Source: CAD feature listing. Evaluate the final solid. Frame: model axes, mm. Face numbers are marked on the shaded views. A direction names the side the tool comes from. Give positions to 0.01 mm unless a question says otherwise; leave off trailing zeros. Loops run counter-clockwise (first coordinate to the right, second up) from the corner with the lowest first, then second, coordinate; pieces in that order, holes last. Notation, with made-up numbers: M -33.75,6.5 L -3.75,6.5 A23 cw -3.75,29.5 Z; hole C -38,7.25 d5. An arc over 180 degrees is marked long. Answer in a Markdown table with one row per item.
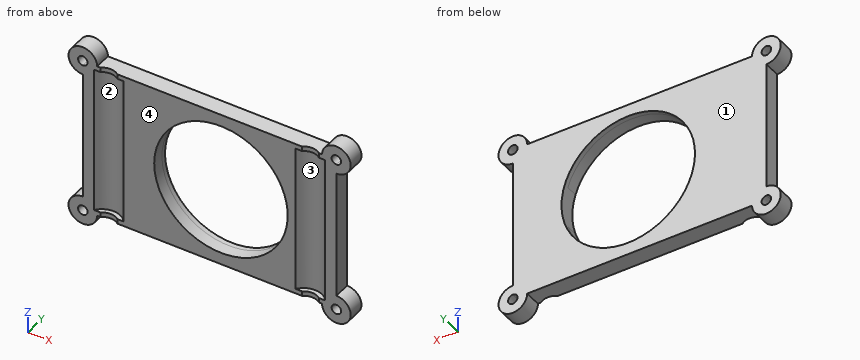
```python
from build123d import *
from build123d.topology import SkipClean

# Parameters (mm, degrees)
SKETCH1_W               = 21.76
SKETCH1_H               = 66
SKETCH1_W_2             = 62.8
BOSS_EXTRUDE1_DEPTH     = 10
SKETCH1_5_W             = 62.8
SKETCH1_5_H             = 66
CUT_EXTRUDE1_DEPTH      = 5
SKETCH3_R               = 7.65
SKETCH3_R_2             = 5.75
CUT_EXTRUDE2_DEPTH      = 62
CUT_EXTRUDE3_DEPTH      = 84.797288739
CUT_EXTRUDE3_DEPTH_BACK = 84.797288739
SKETCH3_3_R             = 5.75
BOSS_EXTRUDE2_DEPTH     = 10
CUT_EXTRUDE4_DEPTH      = 72.560503073
SKETCH5_R               = 28
CUT_EXTRUDE5_DEPTH      = 72.560503073
BOSS_EXTRUDE3_DEPTH     = 5
CUT_EXTRUDE6_START      = -3
CUT_EXTRUDE6_DEPTH      = 3


with BuildPart() as part:
    # Sketch1 → Boss-Extrude1 (new body)
    with BuildSketch(Plane(origin=(0, 0, 0), x_dir=(1, 0, 0), z_dir=(0, 1, 0))):
        with Locations((-42.28, 0)):
            Rectangle(SKETCH1_W, SKETCH1_H)
        Rectangle(SKETCH1_W_2, SKETCH1_H)
        with Locations((42.28, 0)):
            Rectangle(SKETCH1_W, SKETCH1_H)
    extrude(amount=BOSS_EXTRUDE1_DEPTH)

    # Sketch1<5> → Cut-Extrude1 (cut)
    with BuildSketch(Plane(origin=(0, 0, 0), x_dir=(1, 0, 0), z_dir=(0, 1, 0))):
        Rectangle(SKETCH1_5_W, SKETCH1_5_H)
    extrude(amount=CUT_EXTRUDE1_DEPTH, mode=Mode.SUBTRACT)

    # Sketch3 → Cut-Extrude2 (cut)
    # profile 1 of 4: a face of its own
    with BuildSketch(Plane.XY.offset(31)):
        with Locations((-42.25, -4.5)):
            Circle(SKETCH3_R)
        with Locations((-42.25, -4.5)):
            Circle(SKETCH3_R_2, mode=Mode.SUBTRACT)
    # profile 2 of 4: a face of its own
    with BuildSketch(Plane.XY.offset(31)):
        with Locations((-42.25, -4.5)):
            Circle(SKETCH3_R_2)
    # profile 3 of 4: a face of its own
    with BuildSketch(Plane.XY.offset(31)):
        with Locations((42.31, -4.5)):
            Circle(SKETCH3_R)
        with Locations((42.31, -4.5)):
            Circle(SKETCH3_R_2, mode=Mode.SUBTRACT)
    # profile 4 of 4: a face of its own
    with BuildSketch(Plane.XY.offset(31)):
        with Locations((42.31, -4.5)):
            Circle(SKETCH3_R_2)
    extrude(amount=-CUT_EXTRUDE2_DEPTH, mode=Mode.SUBTRACT)

    # Sketch3<3> → Cut-Extrude3 (cut, two sides: drawn at the far end of the back side and taken through both)
    with BuildSketch(Plane.XY.offset(31).offset(-CUT_EXTRUDE3_DEPTH_BACK)):
        with Locations((42.31, -4.5)):
            Circle(SKETCH3_3_R)
        with Locations((-42.25, -4.5)):
            Circle(SKETCH3_3_R)
    extrude(amount=CUT_EXTRUDE3_DEPTH + CUT_EXTRUDE3_DEPTH_BACK, mode=Mode.SUBTRACT)

    # Sketch4 → Boss-Extrude2 (add)
    with BuildSketch(Plane.XZ):
        with BuildLine():
            Line((-51.16, 33), (-47.16, 33))
            ThreePointArc((-47.16, 33), (-57.402640687, 37.242640687), (-53.16, 27))
            Line((-53.16, 27), (-53.16, 31))
            ThreePointArc((-53.16, 31), (-54.574213562, 34.414213562), (-51.16, 33))
        make_face()
        with BuildLine():
            ThreePointArc((-53.16, -27), (-57.402640687, -37.242640687), (-47.16, -33))
            Line((-47.16, -33), (-51.16, -33))
            ThreePointArc((-51.16, -33), (-54.574213562, -34.414213562), (-53.16, -31))
            Line((-53.16, -31), (-53.16, -27))
        make_face()
        with BuildLine():
            ThreePointArc((47.16, -33), (57.402640687, -37.242640687), (53.16, -27))
            Line((53.16, -27), (53.16, -31))
            ThreePointArc((53.16, -31), (54.574213562, -34.414213562), (51.16, -33))
            Line((51.16, -33), (47.16, -33))
        make_face()
        with BuildLine():
            ThreePointArc((53.16, 27), (57.402640687, 37.242640687), (47.16, 33))
            Line((47.16, 33), (51.16, 33))
            ThreePointArc((51.16, 33), (54.574213562, 34.414213562), (53.16, 31))
            Line((53.16, 31), (53.16, 27))
        make_face()
    extrude(amount=-BOSS_EXTRUDE2_DEPTH)

    # Sketch4<3> → Cut-Extrude4 (cut, through all)
    with SkipClean():  # the faces are left unmerged after this step: merging them gives an invalid solid
        with BuildSketch(Plane.XZ):
            with BuildLine():
                ThreePointArc((51.16, 33), (51.745786438, 31.585786438), (53.16, 31))
                Line((53.16, 31), (53.16, 33))
                Line((53.16, 33), (51.16, 33))
            make_face()
            with BuildLine():
                Line((53.16, 33), (53.16, 31))
                ThreePointArc((53.16, 31), (54.574213562, 31.585786438), (55.16, 33))
                ThreePointArc((55.16, 33), (53.16, 35), (51.16, 33))
                Line((51.16, 33), (53.16, 33))
            make_face()
            with BuildLine():
                ThreePointArc((55.16, -33), (54.574213562, -31.585786438), (53.16, -31))
                Line((53.16, -31), (53.16, -33))
                Line((53.16, -33), (51.16, -33))
                ThreePointArc((51.16, -33), (53.16, -35), (55.16, -33))
            make_face()
            with BuildLine():
                Line((53.16, -33), (53.16, -31))
                ThreePointArc((53.16, -31), (51.745786438, -31.585786438), (51.16, -33))
                Line((51.16, -33), (53.16, -33))
            make_face()
            with BuildLine():
                ThreePointArc((-53.16, -31), (-54.574213562, -34.414213562), (-51.16, -33))
                Line((-51.16, -33), (-53.16, -33))
                Line((-53.16, -33), (-53.16, -31))
            make_face()
            with BuildLine():
                Line((-53.16, -33), (-51.16, -33))
                ThreePointArc((-51.16, -33), (-51.745786438, -31.585786438), (-53.16, -31))
                Line((-53.16, -31), (-53.16, -33))
            make_face()
            with BuildLine():
                ThreePointArc((-53.16, 31), (-51.745786438, 31.585786438), (-51.16, 33))
                Line((-51.16, 33), (-53.16, 33))
                Line((-53.16, 33), (-53.16, 31))
            make_face()
            with BuildLine():
                Line((-53.16, 33), (-51.16, 33))
                ThreePointArc((-51.16, 33), (-54.574213562, 34.414213562), (-53.16, 31))
                Line((-53.16, 31), (-53.16, 33))
            make_face()
        extrude(amount=-CUT_EXTRUDE4_DEPTH, mode=Mode.SUBTRACT)

    # Sketch5 → Cut-Extrude5 (cut, through all)
    with SkipClean():  # the faces are left unmerged after this step: merging them gives an invalid solid
        with BuildSketch(Plane(origin=(0, 10, 0), x_dir=(1, 0, 0), z_dir=(0, 1, 0))):
            with Locations(Location((4.77, 0, 0), (0, 0, 270))):
                Circle(SKETCH5_R)
        extrude(amount=-CUT_EXTRUDE5_DEPTH, mode=Mode.SUBTRACT)

    # Sketch6 → Boss-Extrude3 (add)
    with SkipClean():  # the faces are left unmerged after this step: merging them gives an invalid solid
        with BuildSketch(Plane.XZ.offset(-5)):
            with BuildLine():
                Line((31.4, -33), (31.4, -8.651190669))
                ThreePointArc((31.4, -8.651190669), (-23.23, 0), (31.4, 8.651190669))
                Line((31.4, 8.651190669), (31.4, 33))
                Line((31.4, 33), (-31.4, 33))
                Line((-31.4, 33), (-31.4, -33))
                Line((-31.4, -33), (31.4, -33))
            make_face()
        extrude(amount=BOSS_EXTRUDE3_DEPTH)

    # Sketch8 → Cut-Extrude6 (cut)
    with SkipClean():  # the faces are left unmerged after this step: merging them gives an invalid solid
        with BuildSketch(Plane(origin=(0, 10, 0), x_dir=(1, 0, 0), z_dir=(0, 1, 0)).offset(CUT_EXTRUDE6_START)):
            with BuildLine():
                Line((-53.16, 27), (-53.16, -27))
                ThreePointArc((-53.16, -27), (-57.402640687, -37.242640687), (-47.16, -33))
                Line((-47.16, -33), (47.16, -33))
                ThreePointArc((47.16, -33), (57.402640687, -37.242640687), (53.16, -27))
                Line((53.16, -27), (53.16, 27))
                ThreePointArc((53.16, 27), (57.402640687, 37.242640687), (47.16, 33))
                Line((47.16, 33), (-47.16, 33))
                ThreePointArc((-47.16, 33), (-57.402640687, 37.242640687), (-53.16, 27))
            make_face()
        extrude(amount=CUT_EXTRUDE6_DEPTH, mode=Mode.SUBTRACT)


solid = part.part
```
Q1. Reachability of the marked faces 3 and 4 from +Z, -Z, +X, -X, +Y, -Y: full face, straight path, thin tool, end or side. Return the list, or none.
Values follow:
| item | result |
|---|---|
| face 3 | -Y |
| face 4 | +Z, -Z, +X, -X, -Y |
Q2. Section query B-B (x = 4.77). Output: boundary loops of the cut face in (y, z).
Values follow:
| item | result |
|---|---|
| outline | M 0,-33 L 7,-33 L 7,-28 L 0,-28 Z; M 0,28 L 7,28 L 7,33 L 0,33 Z |
Q3. Mould query, pull axis X, two halves, no side actions, for the marked faces 1 and 2. Classes: +X half, -X half, draft (parallel to the pull), parting line (faces both ways), or undercut.
Values follow:
| item | result |
|---|---|
| face 1 | draft |
| face 2 | undercut |
Q4. Ray query, probe 1 along Z at (x, y) = (4.77, 3); probe 2 along X at (y, z) = (4.25, 33.5); probe 3 along Z at (x, y) = (-51.5, 2.25). Return the intervals inside material, ascending. Write a range as from..to.
Values follow:
| item | result |
|---|---|
| probe 1 | -33..-28, 28..33 |
| probe 2 | -59.14..-55.1, -51.22..-47.18, 47.18..51.22, 55.1..59.14 |
| probe 3 | -38.77..-34.12, -31.88..31.88, 34.12..38.77 |
Q5. Section query D-D (x = -8.5). Output: boundary loops of the cut face in (y, z).
Values follow:
| item | result |
|---|---|
| outline | M 0,-33 L 7,-33 L 7,-24.66 L 0,-24.66 Z; M 0,24.66 L 7,24.66 L 7,33 L 0,33 Z |
Q6. Section query A-A (z = 0). Output: boundary loops of the cut face in (x, y).
Values follow:
| item | result |
|---|---|
| outline | M -53.16,0 L -48.44,0 A7.65 cw -36.06,0 L -23.23,0 L -23.23,7 L -53.16,7 Z; M 32.77,0 L 36.12,0 A7.65 cw 48.5,0 L 53.16,0 L 53.16,7 L 32.77,7 Z |
Q7. Contact query for flat-ended pins moving along their axis: pin 1 Ø1.5 at (x, z) = (-37, -8) entering from -Y; pin 2 Ø3.5 at (x, z) = (-53.16, -33) entering from -Y; pin 3 Ø2.5 at (x, y) = (42.5, 2) entering from +Z; pin 4 Ø1 at (y, z) = (1.5, 2) entering from +X. Output: stop coordinate, or through.
Values follow:
| item | result |
|---|---|
| pin 1 | y = 0.25 |
| pin 2 | through |
| pin 3 | z = 33 |
| pin 4 | x = 53.16 |
Q8. Section query C-C (z = 16.5). Output: boundary loops of the cut face in (x, y).
Values follow:
| item | result |
|---|---|
| outline | M -53.16,0 L -48.44,0 A7.65 cw -36.06,0 L -17.85,0 L -17.85,7 L -53.16,7 Z; M 27.39,0 L 36.12,0 A7.65 cw 48.5,0 L 53.16,0 L 53.16,7 L 27.39,7 Z |
